from build123d import *

# Parameters (mm, degrees)
F0_R      = 7.5
F1_DEPTH  = 25
F2_W      = 3
F2_H      = 3
F3_DEPTH  = 60
F3_FACE_W = 3
F3_FACE_H = 3


with BuildPart() as f1:
    # F0 (on Top) → F1 (new body)
    with BuildSketch(Plane.XY):
        Circle(F0_R)
    extrude(amount=F1_DEPTH)

    # F2 (on face) → F3 (join)
    with BuildSketch(Plane.XY.offset(25)):
        Rectangle(F2_W, F2_H)
    extrude(amount=F3_DEPTH)

    # F3_face (on face) → F5 section 0
    with BuildSketch(Plane.XY.offset(85), mode=Mode.PRIVATE) as f5_s0:
        Rectangle(F3_FACE_W, F3_FACE_H)
    loft([f5_s0.sketch, Vertex(0, 0, 90)])


solid = f1.part
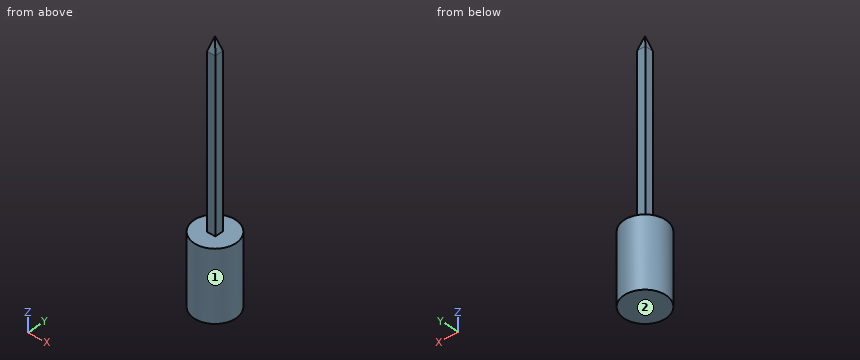
CAD build for the part. Positions are in the model's coordinates, mm. Face numbers are marked on the shaded views. Give positions to 0.01 mm unless a question says otherwise; leave off trailing zeros. Write each loop counter-clockwise with the first axis right and the second up, starting at its lowest first coordinate (ties: lowest second). Pieces come first, ordered by that corner, then holes. Notation, with made-up numbers: (70, 79) - (98, 79) arc R27 cw to (98, 114) - close; hole circle Ø6 at (73.5, 71). An arc over 180 degrees is marked (long way). Put each result on its own line as item: value.
(1) Saw through at D-D (z = 81). List the corners of the cut face in (x, y).
Working result:
outline: (-1.5, -1.5) - (1.5, -1.5) - (1.5, 1.5) - (-1.5, 1.5) - close
(2) Saw through at C-C (x = 4.5). List the corners of the cut face in (y, z), then the cut area to 3 significant figures.
Working result:
outline: (-6, 0) - (6, 0) - (6, 25) - (-6, 25) - close
area: 300 mm^2
(3) Saw through at B-B (z = 20). List the corners of the cut face in (x, y), then the cut area to 3 significant figures.
Working result:
outline: circle Ø15 at (0, 0)
area: 177 mm^2
(4) Saw through at A-A (y = 0.75). List the corners of the cut face in (x, z), then the cut area to 3 significant figures.
Working result:
outline: (-7.46, 0) - (7.46, 0) - (7.46, 25) - (1.5, 25) - (1.5, 85) - (0.75, 87.5) - (-0.75, 87.5) - (-1.5, 85) - (-1.5, 25) - (-7.46, 25) - close
area: 559 mm^2
(5) Pull direction Y, two halves, no side cores. Call the marked faces 1 and 2: released by +Y, released by -Y, zero draft, split by the parting line, or undercut.
Working result:
face 1: split by the parting line
face 2: zero draft
(6) Drop flat-ended pins along their axis: pin 1 Ø4 at (x, z) = (0.5, 47) entering from -Y; pin 2 Ø2.5 at (y, z) = (-0.5, 69) entering from -X; pin 3 Ø2.5 at (y, z) = (-0.5, 45.5) entering from +X; pin 4 Ø1 at (x, y) = (-0.5, 3) entering from -Z. Give the stop position or say it passes through.
Working result:
pin 1: y = -1.5
pin 2: x = -1.5
pin 3: x = 1.5
pin 4: z = 0
(7) Wall check: L1, parallel to X at y = 0.75, z = 44; L2, parallel to Z at x = 4.5, y = -1; L3, parallel to Y at x = -3.5, z = 14. Give the ranges that are in metal, low to high.
Working result:
L1: -1.5 to 1.5
L2: 0 to 25
L3: -6.63 to 6.63
